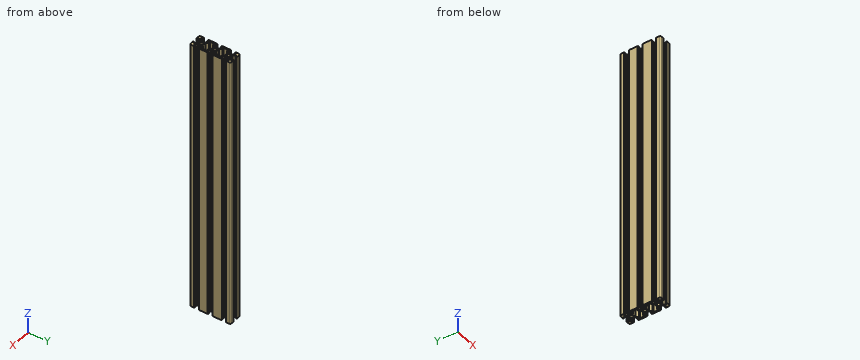
from build123d import *

# Parameters (mm, degrees)
SKETCH_28_R     = 2.5
EXTRUDE_1_DEPTH = 407


with BuildPart() as part:
    # 草图28 → 凸台-拉伸1 (new body)
    with BuildSketch(Plane.XY):
        with BuildLine():
            Line((9.5, 36.4), (9.5, 36.9))
            Line((9.5, 36.9), (8, 36.9))
            Line((8, 36.9), (8, 34.5))
            Line((8, 34.5), (6.489949494, 34.5))
            Line((6.489949494, 34.5), (3.9, 37.089949494))
            Line((3.9, 37.089949494), (3.9, 39.480384758))
            Line((3.9, 39.480384758), (3.6, 40))
            Line((3.6, 40), (3.9, 40.519615242))
            Line((3.9, 40.519615242), (3.9, 42.910050506))
            Line((3.9, 42.910050506), (6.489949494, 45.5))
            Line((6.489949494, 45.5), (8, 45.5))
            Line((8, 45.5), (8, 43.1))
            Line((8, 43.1), (9.5, 43.1))
            Line((9.5, 43.1), (9.5, 43.6))
            Line((9.5, 43.6), (10, 43.6))
            Line((10, 43.6), (10, 48.5))
            ThreePointArc((10, 48.5), (9.560660172, 49.560660172), (8.5, 50))
            Line((8.5, 50), (3.6, 50))
            Line((3.6, 50), (3.6, 49.5))
            Line((3.6, 49.5), (3.1, 49.5))
            Line((3.1, 49.5), (3.1, 48))
            Line((3.1, 48), (5.5, 48))
            Line((5.5, 48), (5.5, 46.489949494))
            Line((5.5, 46.489949494), (2.910050506, 43.9))
            Line((2.910050506, 43.9), (0.519615242, 43.9))
            Line((0.519615242, 43.9), (0, 43.6))
            Line((0, 43.6), (-0.519615242, 43.9))
            Line((-0.519615242, 43.9), (-2.910050506, 43.9))
            Line((-2.910050506, 43.9), (-5.5, 46.489949494))
            Line((-5.5, 46.489949494), (-5.5, 48))
            Line((-5.5, 48), (-3.1, 48))
            Line((-3.1, 48), (-3.1, 49.5))
            Line((-3.1, 49.5), (-3.6, 49.5))
            Line((-3.6, 49.5), (-3.6, 50))
            Line((-3.6, 50), (-8.5, 50))
            ThreePointArc((-8.5, 50), (-9.560660172, 49.560660172), (-10, 48.5))
            Line((-10, 48.5), (-10, 43.6))
            Line((-10, 43.6), (-9.5, 43.6))
            Line((-9.5, 43.6), (-9.5, 43.1))
            Line((-9.5, 43.1), (-8, 43.1))
            Line((-8, 43.1), (-8, 45.5))
            Line((-8, 45.5), (-6.489949494, 45.5))
            Line((-6.489949494, 45.5), (-3.9, 42.910050506))
            Line((-3.9, 42.910050506), (-3.9, 40.519615242))
            Line((-3.9, 40.519615242), (-3.6, 40))
            Line((-3.6, 40), (-3.9, 39.480384758))
            Line((-3.9, 39.480384758), (-3.9, 37.089949494))
            Line((-3.9, 37.089949494), (-6.489949494, 34.5))
            Line((-6.489949494, 34.5), (-8, 34.5))
            Line((-8, 34.5), (-8, 36.9))
            Line((-8, 36.9), (-9.5, 36.9))
            Line((-9.5, 36.9), (-9.5, 36.4))
            Line((-9.5, 36.4), (-10, 36.4))
            Line((-10, 36.4), (-10, 23.6))
            Line((-10, 23.6), (-9.5, 23.6))
            Line((-9.5, 23.6), (-9.5, 23.1))
            Line((-9.5, 23.1), (-8, 23.1))
            Line((-8, 23.1), (-8, 25.5))
            Line((-8, 25.5), (-6.489949494, 25.5))
            Line((-6.489949494, 25.5), (-3.9, 22.910050506))
            Line((-3.9, 22.910050506), (-3.9, 20.519615242))
            Line((-3.9, 20.519615242), (-3.6, 20))
            Line((-3.6, 20), (-3.9, 19.480384758))
            Line((-3.9, 19.480384758), (-3.9, 17.089949494))
            Line((-3.9, 17.089949494), (-6.489949494, 14.5))
            Line((-6.489949494, 14.5), (-8, 14.5))
            Line((-8, 14.5), (-8, 16.9))
            Line((-8, 16.9), (-9.5, 16.9))
            Line((-9.5, 16.9), (-9.5, 16.4))
            Line((-9.5, 16.4), (-10, 16.4))
            Line((-10, 16.4), (-10, 3.6))
            Line((-10, 3.6), (-9.5, 3.6))
            Line((-9.5, 3.6), (-9.5, 3.1))
            Line((-9.5, 3.1), (-8, 3.1))
            Line((-8, 3.1), (-8, 5.5))
            Line((-8, 5.5), (-6.489949494, 5.5))
            Line((-6.489949494, 5.5), (-3.9, 2.910050506))
            Line((-3.9, 2.910050506), (-3.9, 0.519615242))
            Line((-3.9, 0.519615242), (-3.6, 0))
            Line((-3.6, 0), (-3.9, -0.519615242))
            Line((-3.9, -0.519615242), (-3.9, -2.910050506))
            Line((-3.9, -2.910050506), (-6.489949494, -5.5))
            Line((-6.489949494, -5.5), (-8, -5.5))
            Line((-8, -5.5), (-8, -3.1))
            Line((-8, -3.1), (-9.5, -3.1))
            Line((-9.5, -3.1), (-9.5, -3.6))
            Line((-9.5, -3.6), (-10, -3.6))
            Line((-10, -3.6), (-10, -8.5))
            ThreePointArc((-10, -8.5), (-9.560660172, -9.560660172), (-8.5, -10))
            Line((-8.5, -10), (-3.6, -10))
            Line((-3.6, -10), (-3.6, -9.5))
            Line((-3.6, -9.5), (-3.1, -9.5))
            Line((-3.1, -9.5), (-3.1, -8))
            Line((-3.1, -8), (-5.5, -8))
            Line((-5.5, -8), (-5.5, -6.489949494))
            Line((-5.5, -6.489949494), (-2.910050506, -3.9))
            Line((-2.910050506, -3.9), (-0.519615242, -3.9))
            Line((-0.519615242, -3.9), (0, -3.6))
            Line((0, -3.6), (0.519615242, -3.9))
            Line((0.519615242, -3.9), (2.910050506, -3.9))
            Line((2.910050506, -3.9), (5.5, -6.489949494))
            Line((5.5, -6.489949494), (5.5, -8))
            Line((5.5, -8), (3.1, -8))
            Line((3.1, -8), (3.1, -9.5))
            Line((3.1, -9.5), (3.6, -9.5))
            Line((3.6, -9.5), (3.6, -10))
            Line((3.6, -10), (8.5, -10))
            ThreePointArc((8.5, -10), (9.560660172, -9.560660172), (10, -8.5))
            Line((10, -8.5), (10, -3.6))
            Line((10, -3.6), (9.5, -3.6))
            Line((9.5, -3.6), (9.5, -3.1))
            Line((9.5, -3.1), (8, -3.1))
            Line((8, -3.1), (8, -5.5))
            Line((8, -5.5), (6.489949494, -5.5))
            Line((6.489949494, -5.5), (3.9, -2.910050506))
            Line((3.9, -2.910050506), (3.9, -0.519615242))
            Line((3.9, -0.519615242), (3.6, 0))
            Line((3.6, 0), (3.9, 0.519615242))
            Line((3.9, 0.519615242), (3.9, 2.910050506))
            Line((3.9, 2.910050506), (6.489949494, 5.5))
            Line((6.489949494, 5.5), (8, 5.5))
            Line((8, 5.5), (8, 3.1))
            Line((8, 3.1), (9.5, 3.1))
            Line((9.5, 3.1), (9.5, 3.6))
            Line((9.5, 3.6), (10, 3.6))
            Line((10, 3.6), (10, 16.4))
            Line((10, 16.4), (9.5, 16.4))
            Line((9.5, 16.4), (9.5, 16.9))
            Line((9.5, 16.9), (8, 16.9))
            Line((8, 16.9), (8, 14.5))
            Line((8, 14.5), (6.489949494, 14.5))
            Line((6.489949494, 14.5), (3.9, 17.089949494))
            Line((3.9, 17.089949494), (3.9, 19.480384758))
            Line((3.9, 19.480384758), (3.6, 20))
            Line((3.6, 20), (3.9, 20.519615242))
            Line((3.9, 20.519615242), (3.9, 22.910050506))
            Line((3.9, 22.910050506), (6.489949494, 25.5))
            Line((6.489949494, 25.5), (8, 25.5))
            Line((8, 25.5), (8, 23.1))
            Line((8, 23.1), (9.5, 23.1))
            Line((9.5, 23.1), (9.5, 23.6))
            Line((9.5, 23.6), (10, 23.6))
            Line((10, 23.6), (10, 36.4))
            Line((10, 36.4), (9.5, 36.4))
        make_face()
        Circle(SKETCH_28_R, mode=Mode.SUBTRACT)
        with Locations((0, 20)):
            Circle(SKETCH_28_R, mode=Mode.SUBTRACT)
        with Locations((0, 40)):
            Circle(SKETCH_28_R, mode=Mode.SUBTRACT)
        Polygon((2.910050506, 16.1), (5.910050506, 13.1), (8, 13.1), (8, 6.9), (5.910050506, 6.9), (2.910050506, 3.9), (-2.910050506, 3.9), (-5.910050506, 6.9), (-8, 6.9), (-8, 13.1), (-5.910050506, 13.1), (-2.910050506, 16.1), align=None, mode=Mode.SUBTRACT)
        Polygon((5.910050506, 26.9), (2.910050506, 23.9), (-2.910050506, 23.9), (-5.910050506, 26.9), (-8, 26.9), (-8, 33.1), (-5.910050506, 33.1), (-2.910050506, 36.1), (2.910050506, 36.1), (5.910050506, 33.1), (8, 33.1), (8, 26.9), align=None, mode=Mode.SUBTRACT)
    extrude(amount=EXTRUDE_1_DEPTH)


solid = part.part
Work out the finished part from the listing and answer in its coordinate system (mm). Round coordinates to 2 decimals unless told otherwise and drop trailing zeros.
1) Straight lines are drawn through the part: line 1 (Y direction, x = 0.5, z = 227); line 2 (Y direction, x = 0, z = 128); line 3 (X direction, y = 0.5, z = 379.5). For each, find the intervals that lie inside material, in ascending order.
2) Given pin 1 Ø3 at (x, z) = (-0.5, 106.5) entering from +Y; pin 2 Ø1.9 at (y, z) = (1.5, 179.5) entering from +X; pin 3 Ø1.9 at (y, z) = (21.5, 269.5) entering from -X, each flat-ended and moving along its own axis, determine where each tip first touches the part or whether it passes through.
3) A cutting plane is placed at A-A (z = 99.5). Give the number of separate pieces and of enclosed holes in the cut face, plus the area to 3 significant figures.
Completed:
1. line 1: y = -3.89 to -2.45, 2.45 to 3.9, 16.1 to 17.55, 22.45 to 23.9, 36.1 to 37.55, 42.45 to 43.89
1. line 2: y = -3.6 to -2.5, 2.5 to 3.9, 16.1 to 17.5, 22.5 to 23.9, 36.1 to 37.5, 42.5 to 43.6
1. line 3: x = -3.89 to -2.45, 2.45 to 3.89
2. pin 1: stops at y = 43.9
2. pin 2: stops at x = 3.9
2. pin 3: stops at x = -3.9
3. separate pieces: 1
3. enclosed holes: 5
3. area: 423 mm2
